Can you work these out from the model? Positions are in its coordinate system, mm. A direction names the side the tool comes from. Give positions to 0.01 mm unless a question says otherwise; leave off trailing zeros. Write each loop counter-clockwise with the first axis right and the second up, starting at its lowest first coordinate (ties: lowest second). Pieces come first, ordered by that corner, then holes. Notation, with made-up numbers: (71, 36) - (78, 36) arc R26 ccw to (78, 72) - close; hole circle Ø5 at (85, 17). An arc over 180 degrees is marked (long way). Return JSON: item names as keys, results as strings. Group by question number.
from build123d import *

# Parameters (mm, degrees)
CYLINDER018_R     = 1.5
CYLINDER018_DEPTH = 25
CYLINDER020_R     = 2.8
CYLINDER020_DEPTH = 5
CHAMFER001_SIZE   = 2
CYLINDER016_R     = 1.5
CYLINDER016_DEPTH = 25
CYLINDER017_R     = 1.5
CYLINDER017_DEPTH = 25
CYLINDER021_R     = 2.8
CYLINDER021_DEPTH = 5
CHAMFER002_SIZE   = 2
CYLINDER015_R     = 1.5
CYLINDER015_DEPTH = 25
CYLINDER019_R     = 2.8
CYLINDER019_DEPTH = 5
CHAMFER003_SIZE   = 2
BOX018_W          = 40
BOX018_H          = 8
BOX018_DEPTH      = 5
FILLET014_R       = 3.9
CYLINDER022_R     = 2.8
CYLINDER022_DEPTH = 5
CHAMFER_SIZE      = 2
BOX017_W          = 22
BOX017_H          = 18
BOX017_DEPTH      = 8


with BuildPart() as obj1:
    # Cylinder018 → Cylinder018 (new body)
    with BuildSketch(Plane(origin=(25, 24, 2), x_dir=(1, 0, 0), z_dir=(0, 0, 1))):
        Circle(CYLINDER018_R)
    extrude(amount=CYLINDER018_DEPTH)


with BuildPart() as chamfer001:
    # Cylinder020 → Cylinder020 (new body)
    with BuildSketch(Plane(origin=(25, 36, 18), x_dir=(1, 0, 0), z_dir=(0, 0, 1))):
        Circle(CYLINDER020_R)
    extrude(amount=CYLINDER020_DEPTH)

    # Chamfer001
    chamfer001_edges = [chamfer001.edges().sort_by_distance(p)[0] for p in [
        (22.2, 36, 18),
    ]]
    chamfer(chamfer001_edges, length=CHAMFER001_SIZE)


with BuildPart() as obj2:
    # Cylinder016 → Cylinder016 (new body)
    with BuildSketch(Plane(origin=(25, 36, 2), x_dir=(1, 0, 0), z_dir=(0, 0, 1))):
        Circle(CYLINDER016_R)
    extrude(amount=CYLINDER016_DEPTH)


with BuildPart() as obj3:
    # Cylinder017 → Cylinder017 (new body)
    with BuildSketch(Plane(origin=(35, 36, 2), x_dir=(1, 0, 0), z_dir=(0, 0, 1))):
        Circle(CYLINDER017_R)
    extrude(amount=CYLINDER017_DEPTH)


with BuildPart() as chamfer002:
    # Cylinder021 → Cylinder021 (new body)
    with BuildSketch(Plane(origin=(35, 36, 18), x_dir=(1, 0, 0), z_dir=(0, 0, 1))):
        Circle(CYLINDER021_R)
    extrude(amount=CYLINDER021_DEPTH)

    # Chamfer002
    chamfer002_edges = [chamfer002.edges().sort_by_distance(p)[0] for p in [
        (32.2, 36, 18),
    ]]
    chamfer(chamfer002_edges, length=CHAMFER002_SIZE)


with BuildPart() as obj4:
    # Cylinder015 → Cylinder015 (new body)
    with BuildSketch(Plane(origin=(35, 24, 2), x_dir=(1, 0, 0), z_dir=(0, 0, 1))):
        Circle(CYLINDER015_R)
    extrude(amount=CYLINDER015_DEPTH)


with BuildPart() as chamfer003:
    # Cylinder019 → Cylinder019 (new body)
    with BuildSketch(Plane(origin=(35, 24, 18), x_dir=(1, 0, 0), z_dir=(0, 0, 1))):
        Circle(CYLINDER019_R)
    extrude(amount=CYLINDER019_DEPTH)

    # Chamfer003
    chamfer003_edges = [chamfer003.edges().sort_by_distance(p)[0] for p in [
        (32.2, 24, 18),
    ]]
    chamfer(chamfer003_edges, length=CHAMFER003_SIZE)


with BuildPart() as fillet014:
    # Box018 → Box018 (new body)
    with BuildSketch(Plane(origin=(10, 26, 12), x_dir=(1, 0, 0), z_dir=(0, 0, 1))):
        with Locations((20, 4)):
            Rectangle(BOX018_W, BOX018_H)
    extrude(amount=BOX018_DEPTH)

    # Fillet014
    fillet014_edges = [fillet014.edges().sort_by_distance(p)[0] for p in [
        (30, 26, 17),
        (30, 34, 17),
    ]]
    fillet(fillet014_edges, radius=FILLET014_R)


with BuildPart() as fusion005007:
    # Cylinder022 → Cylinder022 (new body)
    with BuildSketch(Plane(origin=(25, 24, 18), x_dir=(1, 0, 0), z_dir=(0, 0, 1))):
        Circle(CYLINDER022_R)
    extrude(amount=CYLINDER022_DEPTH)

    # Chamfer
    chamfer_edges = [fusion005007.edges().sort_by_distance(p)[0] for p in [
        (22.2, 24, 18),
    ]]
    chamfer(chamfer_edges, length=CHAMFER_SIZE)

    # Fusion005007: union obj1, Chamfer001, obj2, obj3, Chamfer002, obj4, Chamfer003, Fillet014
    add(obj1.part)
    add(chamfer001.part)
    add(obj2.part)
    add(obj3.part)
    add(chamfer002.part)
    add(obj4.part)
    add(chamfer003.part)
    add(fillet014.part)


with BuildPart() as cablecap:
    # Box017 → Box017 (new body)
    with BuildSketch(Plane(origin=(19, 21, 13), x_dir=(1, 0, 0), z_dir=(0, 0, 1))):
        with Locations((11, 9)):
            Rectangle(BOX017_W, BOX017_H)
    extrude(amount=BOX017_DEPTH)

    # Cut004: cut Fusion005007
    add(fusion005007.part, mode=Mode.SUBTRACT)


with BuildPart() as cablecap_1:
    # Cut004 placement: moved
    add(cablecap.part.moved(Location((0, 0, 4))))


solid = cablecap_1.part
1) Imagine slicing it at A-A, the plane y = 24. Write out the boundary of the cut face in (x, z).
2) We'd pull the mould along Y, two halves only. Please class faces 1 (the face through (23.89, 25.01, 19.81)), 2 (the face through (19, 30, 22)), 3 (the face through (30, 21, 21)): pulls with the +Y half, pulls with the -Y half, needs draft (parallel to the pull), parting line crosses it, or undercut.
3) Imagine slicing it at C-C, the plane z = 21.25. Write out the boundary of the cut face in (x, y), and give its area (3 significant figures).
4) Imagine slicing it at D-D, the plane y = 28. Write out the boundary of the cut face in (x, z).
5) I need wall thicknesses on line 1 along X through (y, z) = (36, 24.85); line 2 along X through (y, z) = (24, 20.7); line 3 along Y through (x, z) = (25, 24.4). Which ranges of each line are inside material? Lowest first, please.
6) Will these pins go through, and if not, where does the flat tip stop? pin 1 Ø1.5 at (y, z) = (32.5, 18.5) entering from -X; pin 2 Ø3.5 at (x, y) = (35, 24) entering from +Z.
7) Imagine slicing it at B-B, the plane x = 25. Write out the boundary of the cut face in (y, z), and give its area (3 significant figures).
8) On a 3-axis mill with a long thin cutter (end or side, diameter ignored), from which of +Z, -Z, +X, -X, +Y, -Y can I reach the whole of each face in a straight line? I mean faces 4 (the face through (30.154, 32.888, 19.827)), 5 (the face through (33.8, 35.1, 19.8)), 6 (the face through (34.393, 33.267, 24.493)). Say none if no direction works.
Resolved:
{
 "1": {"outline": "(19, 17) - (23.5, 17) - (23.5, 22.7) - (22.2, 24) - (22.2, 25) - (19, 25) - close; (26.5, 17) - (33.5, 17) - (33.5, 22.7) - (32.2, 24) - (32.2, 25) - (27.8, 25) - (27.8, 24) - (26.5, 22.7) - close; (36.5, 17) - (41, 17) - (41, 25) - (37.8, 25) - (37.8, 24) - (36.5, 22.7) - close"},
 "2": {"face 1": "undercut", "face 2": "needs draft", "face 3": "pulls with the -Y half"},
 "3": {"outline": "(19, 21) - (41, 21) - (41, 39) - (19, 39) - close; hole circle Ø3 at (25, 24); hole circle Ø3 at (25, 36); hole circle Ø3 at (35, 24); hole circle Ø3 at (35, 36)", "area": "368 mm^2"},
 "4": {"outline": "(19, 20.51) - (41, 20.51) - (41, 25) - (19, 25) - close"},
 "5": {"line 1": "19 to 22.2, 27.8 to 32.2, 37.8 to 41", "line 2": "19 to 23.5, 26.5 to 33.5, 36.5 to 41", "line 3": "21 to 21.2, 26.8 to 33.2, 38.8 to 39"},
 "6": {"pin 1": "through", "pin 2": "z = 22.95"},
 "7": {"outline": "(21, 17) - (22.5, 17) - (22.5, 22.7) - (21.2, 24) - (21.2, 25) - (21, 25) - close; (25.5, 17) - (26, 17) - (26, 17.1) arc R3.9 cw to (29.9, 21) - (30.1, 21) arc R3.9 cw to (34, 17.1) - (34, 17) - (34.5, 17) - (34.5, 22.7) - (33.2, 24) - (33.2, 25) - (26.8, 25) - (26.8, 24) - (25.5, 22.7) - close; (37.5, 17) - (39, 17) - (39, 25) - (38.8, 25) - (38.8, 24) - (37.5, 22.7) - close", "area": "61.9 mm^2"},
 "8": {"face 4": "-Z, +X, -X", "face 5": "+Z, -Z", "face 6": "+Z"}
}
